Verification items for this drawing (mm, ordinates from the low corner). Round coordinates to 2 decimals unless told otherwise and drop trailing zeros. Loops run counter-clockwise (first coordinate to the right, second up) from the corner with the lowest first, then second, coordinate; pieces in that order, holes last. Notation, with made-up numbers: M -15.75,-14.75 L 2.25,-14.75 A23 ccw 2.25,16.25 Z; hole C 5,88 d8. An arc over 180 degrees is marked long. Write item = value, one per line. Start each with the question number.
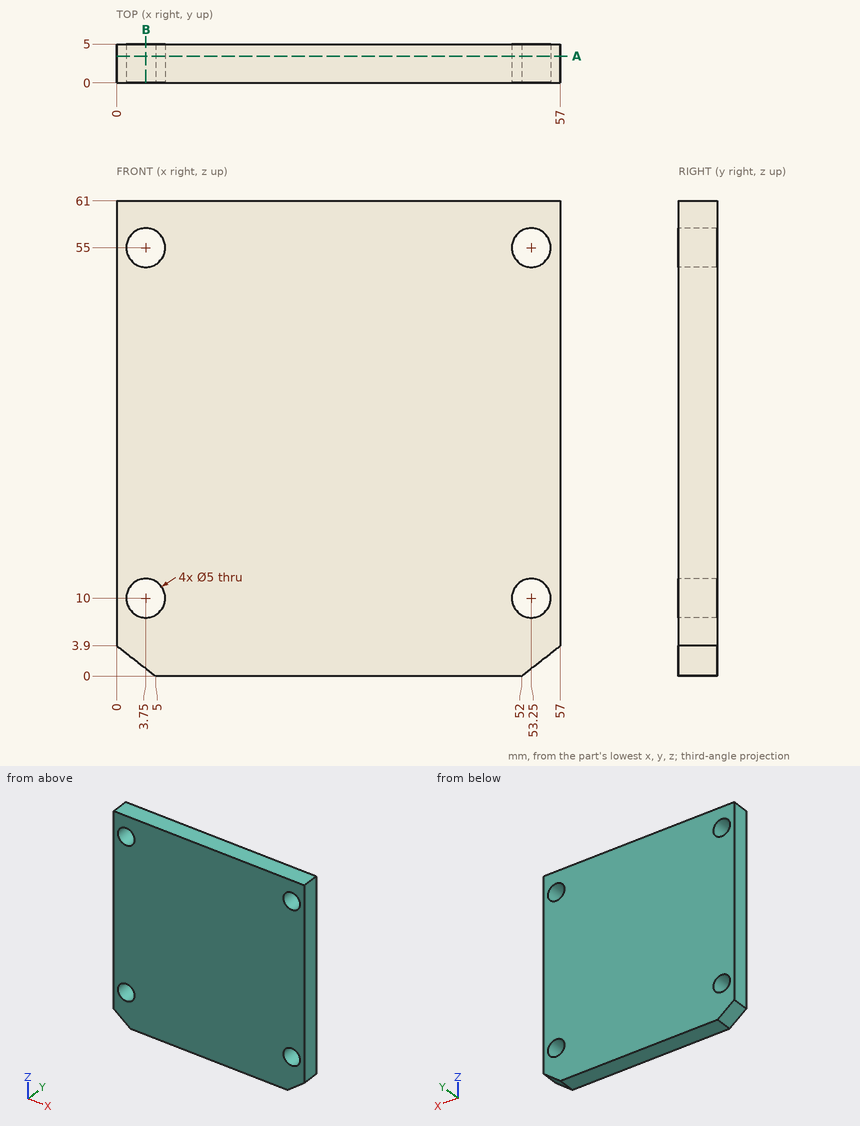
1. Section check A-A, the plane y = 3.45. Enter the section's corners in (x, z), and give its area (3 significant figures).
2. Thickness scan on line 1 (Z direction, x = 4, y = 1.8); line 2 (X direction, y = 1.35, z = 54); line 3 (X direction, y = 1.9, z = 12). Record the ranges inside material, lowest first.
3. Section check B-B, the plane x = 3.75. Enter the section's corners in (y, z) (3 decimals), and give its area (3 significant figures).
Computed values:
q1.outline = M 0,3.9 L 5,0 L 52,0 L 57,3.9 L 57,61 L 0,61 Z; hole C 3.75,10 d5; hole C 3.75,55 d5; hole C 53.25,10 d5; hole C 53.25,55 d5
q1.area = 3,380 mm2
q2.line_1 = 0.78 to 7.51, 12.49 to 52.51, 57.49 to 61
q2.line_2 = 0 to 1.46, 6.04 to 50.96, 55.54 to 57
q2.line_3 = 0 to 2.25, 5.25 to 51.75, 54.75 to 57
q3.outline = M 0,0.975 L 5,0.975 L 5,7.5 L 0,7.5 Z; M 0,12.5 L 5,12.5 L 5,52.5 L 0,52.5 Z; M 0,57.5 L 5,57.5 L 5,61 L 0,61 Z
q3.area = 250 mm2
